from build123d import *

# Parameters (mm, degrees)
F0_W     = 25.4
F0_H     = 58.92757
F1_DEPTH = 25.4
F2_R     = 5.08


with BuildPart() as f1:
    # F0 (on Front) → F1 (new body)
    with BuildSketch(Plane.XZ):
        with Locations((0.082556, 29.463785)):
            Rectangle(F0_W, F0_H)
        Polygon((12.782556, 0), (-12.617444, 0), (-26.336173, -21.37654), (26.501286, -21.37654), align=None)
    extrude(amount=F1_DEPTH)

    # F2
    f2_edges = [f1.edges().sort_by_distance(p)[0] for p in [
        (-19.476808, -25.4, -10.68827),
        (0.082556, -25.4, -21.37654),
        (19.641921, -25.4, -10.68827),
    ]]
    fillet(f2_edges, radius=F2_R)


solid = f1.part
Input: part model. Units: mm. Frame: model coordinates. Give positions to 0.01 mm unless a question says otherwise; leave off trailing zeros. Order: outer loops, then holes, each group sorted by start corner. A loop starts at its lowest first (then second) coordinate and runs counter-clockwise, first axis right, second up. Notation, with made-up numbers: M 32,86 L 42,86 A12 cw 42,94 Z; hole C 4.25,36.25 d7. An arc over 180 degrees is marked long. Answer as a JSON object with one key per item and string values.
1. Cut plane B-B, the plane z = 32.5. Output: boundary loops of the cut face in (x, y), and give its area (3 significant figures).
Result sheet:
{"outline": "M -12.62,-25.4 L 12.78,-25.4 L 12.78,0 L -12.62,0 Z", "area": "645 mm²"}
2. Ray query, line 1 (X direction, y = -4.25, z = 7); line 2 (Z direction, x = 14, y = -10.25); line 3 (Z direction, x = 20, y = -20.5). Return the intervals inside material, ascending. Write a range as [from, to].
Result sheet:
{"line 1": "[-12.62, 12.78]", "line 2": "[-21.38, -1.9]", "line 3": "[-21.37, -11.25]"}
3. First-contact query: P1, Ø10, axis at y = -22.5, z = 13.5, coming from the -X side; P2, Ø7.5, axis at y = -6.5, z = 18.5, coming from the +X side; P3, Ø8, axis at y = -6, z = -11, coming from the -X side. Flat tips, straight axial feed; report the tip coordinate or a pass-through.
Result sheet:
{"P1": "x = -12.62", "P2": "x = 12.78", "P3": "x = -22.24"}
4. Cut plane A-A, the plane y = -19.25. Output: boundary loops of the cut face in (x, z), and give its area (3 significant figures).
Result sheet:
{"outline": "M -26.34,-21.38 L 26.5,-21.38 L 12.78,0 L 12.78,58.93 L -12.62,58.93 L -12.62,0 Z", "area": "2,330 mm²"}
